Autodesk Inventor part; units mm, degrees
ref_plane "YZ Plane" through (0, 0, 0) normal (1, 0, 0) x (0, 1, 0)
ref_plane "XZ Plane" through (0, 0, 0) normal (0, 1, 0) x (-1, 0, 0)
ref_plane "XY Plane" through (0, 0, 0) normal (0, 0, 1) x (1, 0, 0)
sketch "Sketch1" plane through (0, 0, 0) normal (0, 0, 1) x (1, 0, 0)
  circle A0 centre (0, 0) radius 21.082
  circle A1 centre (0, 0) radius 24.13
  circle A2 centre (0, 0) radius 8.7313
  dimension "d0" = 42.164
  dimension "d1" = 48.26
  dimension "d8" = 17.4625
extrude "Extrusion1" add sketch "Sketch1" along normal blind 19.05 contours A1
extrude "Extrusion2" add sketch "Sketch1" against normal blind 5.08 contours A0 | A1 | A2
fillet "Fillet1" radius 6.35 1 edges at (-24.13, 0, -5.08)
fillet "Fillet2" radius 6.35 1 edges at (-21.082, 0, 0)
extrude "Extrusion3" cut sketch "Sketch1" against normal blind 5.08 contours A2
properties part number "PVC Shooter Conveyor End Cap" material "PVC-Piping"
Here's how the part is built. I have some questions about the finished solid (model axes, mm). A direction names the side the tool comes from. Coordinates: 2 decimals unless noted, no trailing zeros. Write each loop counter-clockwise with the first axis right and the second up, starting at its lowest first coordinate (ties: lowest second). Pieces come first, ordered by that corner, then holes. Notation, with made-up numbers: (70, 9) - (84, 9) arc R24 ccw to (84, 27) - close; hole circle Ø6 at (86, -14). An arc over 180 degrees is marked (long way). One line per item, written item: value.
1) I need wall thicknesses on line 1 along Y through (x, z) = (0, 11.5); line 2 along Z through (x, y) = (3, 11.5); line 3 along Y through (x, z) = (-7.5, 9). Which ranges of each line are inside material? Lowest first, please.
Model answer:
line 1: y = -24.13 to -21.08, 21.08 to 24.13
line 2: z = -5.08 to 0
line 3: y = -22.93 to -19.7, 19.7 to 22.93
2) Suppose I cut it at A-A on z = 12.25. Write out the boundary of the cut face in (x, y).
Model answer:
outline: circle Ø48.26 at (0, 0); hole circle Ø42.16 at (0, 0)
3) I'm going to push flat-ended pins straight in: P1, Ø3, axis at x = -10.5, z = 11.5, coming from the -Y side; P2, Ø4, axis at x = 13, z = 12, coming from the -Y side; P3, Ø1, axis at y = 13, z = 10.5, coming from the -X side; P4, Ø15.5, axis at x = 0, y = 0, coming from the -Z side. Where does each tip first touch, or does it pass through?
Model answer:
P1: stops at y = -22.39
P2: stops at y = -21.48
P3: stops at x = -20.64
P4: passes through
4) We'd pull the mould along Y, two halves only. Please class faces 1 (the flat face through (-0.1, -21.3, 19.05)), 2 (the cylindrical face through (20.11, -6.33, 12.61)), 3 (the cylindrical face through (23.016, -7.248, 10.036)): pulls with the +Y half, pulls with the -Y half, needs draft (parallel to the pull), parting line crosses it, or undercut.
Model answer:
face 1: needs draft
face 2: undercut
face 3: parting line crosses it
5) Suppose I cut it at B-B on z = 5.5. Write out the boundary of the cut face in (x, y).
Model answer:
outline: circle Ø48.26 at (0, 0); hole circle Ø42.05 at (0, 0)
6) On a 3-axis mill with a long thin cutter (end or side, diameter ignored), from which of +Z, -Z, +X, -X, +Y, -Y can I reach the whole of each face in a straight line? I mean faces 4 (the flat face through (8, -4, -5.08)), 5 (the flat face through (6.3, -6.3, 0)). Say none if no direction works.
Model answer:
face 4: -Z, +X, -X, +Y, -Y
face 5: +Z
